Verification items for the finished model (mm, model axes). Face numbers are marked on the shaded views. Round coordinates to 2 decimals unless told otherwise and drop trailing zeros. Write each loop counter-clockwise with the first axis right and the second up, starting at its lowest first coordinate (ties: lowest second). Pieces come first, ordered by that corner, then holes. Notation, with made-up numbers: (1, 10) - (27, 10) arc R18 ccw to (27, 21) - close; hole circle Ø10 at (75, 32.5). An arc over 180 degrees is marked (long way). Answer as a JSON object with one key per item and string values.
```python
from build123d import *

# Parameters (mm, degrees)
SKETCH5_R          = 1.6425
CUT_EXTRUDE1_DEPTH = 50.7
SKETCH6_R          = 1.095
CUT_EXTRUDE2_DEPTH = 70.421071799
CUT_EXTRUDE3_START = -7.395857
SKETCH7_R          = 1.095
CUT_EXTRUDE3_DEPTH = 9.861143
CIRPATTERN1_COUNT  = 4


with BuildPart() as part:
    # Sketch2 → Revolve1 (revolve)
    with BuildSketch(Plane.XY, mode=Mode.PRIVATE) as revolve1_sk:
        Polygon((49.7, 12.7), (49.7, 3.2004), (47.675, 3.2004), (47.675, 0), (35.5, 0), (35.5, 3.175), (37.5, 3.175), (37.5, 12.7), align=None)
    revolve(revolve1_sk.sketch.rotate(Axis((0, 0, 0), (0, 1, 0)), 90), axis=Axis((0, 0, 0), (0, 1, 0)))  # turned: the seam where the file's is

    # Sketch5 → Cut-Extrude1 (cut, through all)
    with BuildSketch(Plane.XY):
        with Locations(Location((0, 6.35, 0), (0, 0, 270))):  # turned: the seam where the file's is
            Circle(SKETCH5_R)
    cut_extrude1 = extrude(amount=-CUT_EXTRUDE1_DEPTH, mode=Mode.SUBTRACT)

    # Sketch6 → Cut-Extrude2 (cut, through all)
    with BuildSketch(Plane(origin=(0, 0, 0), x_dir=(0.809016994, 0, 0.587785252), z_dir=(-0.587785252, 0, 0.809016994))):
        with Locations((0, 5.175)):
            Circle(SKETCH6_R)
    cut_extrude2 = extrude(amount=-CUT_EXTRUDE2_DEPTH, mode=Mode.SUBTRACT)

    # Sketch7 → Cut-Extrude3 (cut)
    with BuildSketch(Plane(origin=(-19.76384492, 19.412976321, -27.202598826), x_dir=(0.809016994, 0, -0.587785252), z_dir=(0.50903696, -0.5, 0.700629269)).offset(CUT_EXTRUDE3_START)):
        with Locations(Location((0, -10.926477372, 0), (0, 0, 180))):  # turned: the seam where the file's is
            Circle(SKETCH7_R)
    cut_extrude3 = extrude(amount=CUT_EXTRUDE3_DEPTH, mode=Mode.SUBTRACT)

    # CirPattern1: Cut-Extrude1, Cut-Extrude2, Cut-Extrude3 ×4 about axis
    cirpattern1_axis = Axis((0, 13.335, 0), (0, -1, 0))
    add([cut_extrude1.rotate(cirpattern1_axis, i * 360 / CIRPATTERN1_COUNT) for i in range(1, CIRPATTERN1_COUNT)], mode=Mode.SUBTRACT)
    add([cut_extrude2.rotate(cirpattern1_axis, i * 360 / CIRPATTERN1_COUNT) for i in range(1, CIRPATTERN1_COUNT)], mode=Mode.SUBTRACT)
    add([cut_extrude3.rotate(cirpattern1_axis, i * 360 / CIRPATTERN1_COUNT) for i in range(1, CIRPATTERN1_COUNT)], mode=Mode.SUBTRACT)


solid = part.part
```
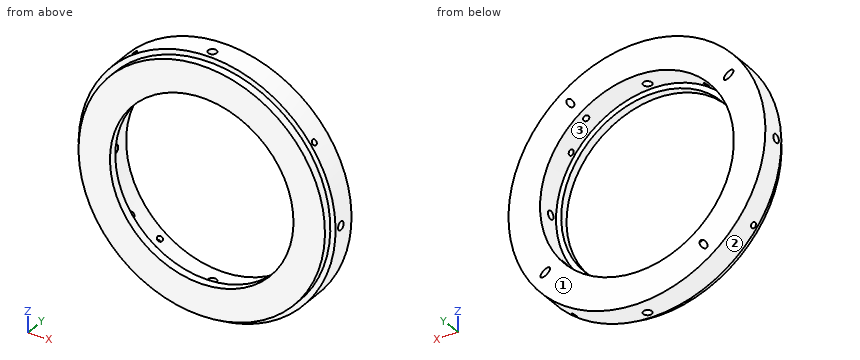
1. Cross-section at D-D (x = -12). Record the boundary of the cut face in (y, z) (3 decimals).
Completed:
{"outline": "(0, -46.14) - (3.2, -46.14) - (3.2, -48.23) - (12.7, -48.23) - (12.7, -35.528) - (3.175, -35.528) - (3.175, -33.41) - (0, -33.41) - close; (0, 33.41) - (3.175, 33.41) - (3.175, 35.528) - (12.7, 35.528) - (12.7, 48.23) - (3.2, 48.23) - (3.2, 46.14) - (0, 46.14) - close"}
2. Cross-section at C-C (z = -18.5). Record the boundary of the cut face in (x, y) (3 decimals).
Completed:
{"outline": "(-46.129, 3.2) - (-43.939, 3.2) - (-43.939, 0) - (-30.299, 0) - (-30.299, 3.175) - (-32.619, 3.175) - (-32.619, 12.7) - (-46.129, 12.7) - close; (30.299, 0) - (43.939, 0) - (43.939, 3.2) - (46.129, 3.2) - (46.129, 12.7) - (32.619, 12.7) - (32.619, 3.175) - (30.299, 3.175) - close"}
3. Go/stop test with flat-tipped pins: pin 1 (22.5 mm diameter, centred on x = 2, z = -13, fed in from +Y); pin 2 (5 mm diameter, centred on y = 1.5, z = 37.5, fed in from -X); pin 3 (5 mm diameter, centred on y = 3.5, z = 4.5, fed in from -X); pin 4 (5 mm diameter, centred on x = 7.5, y = 8, fed in from -Z). Record where each tip stops, or that it passes through.
Completed:
{"pin 1": "passes through", "pin 2": "stops at x = -34.61", "pin 3": "stops at x = -49.66", "pin 4": "stops at z = -49.45"}
4. Mould release check, pull along Z, two halves, no side actions. Record for the marked faces 1, 2 and 3: released by +Z, released by -Z, zero draft, split by the parting line, or undercut.
Completed:
{"face 1": "zero draft", "face 2": "split by the parting line", "face 3": "undercut"}
5. Cross-section at A-A (z = 0). Record the boundary of the cut face in (x, y) (1 decimal), plus the area to 3 significant figures.
Completed:
{"outline": "(-49.7, 3.2) - (-47.7, 3.2) - (-47.7, 0) - (-35.5, 0) - (-35.5, 3.2) - (-37.5, 3.2) - (-37.5, 4.7) - (-49.7, 4.7) - close; (-49.7, 8) - (-37.5, 8) - (-37.5, 12.7) - (-49.7, 12.7) - close; (35.5, 0) - (47.7, 0) - (47.7, 3.2) - (49.7, 3.2) - (49.7, 4.7) - (37.5, 4.7) - (37.5, 3.2) - (35.5, 3.2) - close; (37.5, 8) - (49.7, 8) - (49.7, 12.7) - (37.5, 12.7) - close", "area": "229 mm^2"}
6. Material ranges on probe 1 along X at (y, z) = (9.75, 1.5); probe 2 along X at (y, z) = (2.4, 0) (3 decimals); probe 3 along Z at (x, y) = (-23.5, 6), recorded low to high. Write a range as from..to.
Completed:
{"probe 1": "x = -49.68..-37.47, 37.47..49.68", "probe 2": "x = -47.675..-35.5, 35.5..47.675", "probe 3": "z = -43.79..-29.22, 29.22..31.12, 33.57..43.79"}
7. Cross-section at B-B (x = 0). Record the boundary of the cut face in (y, z) (1 decimal), plus the area to 3 significant figures.
Completed:
{"outline": "(0, -47.7) - (3.2, -47.7) - (3.2, -49.7) - (4.7, -49.7) - (4.7, -37.5) - (3.2, -37.5) - (3.2, -35.5) - (0, -35.5) - close; (0, 35.5) - (3.2, 35.5) - (3.2, 37.5) - (4.7, 37.5) - (4.7, 49.7) - (3.2, 49.7) - (3.2, 47.7) - (0, 47.7) - close; (8, -49.7) - (12.7, -49.7) - (12.7, -37.5) - (8, -37.5) - close; (8, 37.5) - (12.7, 37.5) - (12.7, 49.7) - (8, 49.7) - close", "area": "229 mm^2"}
